The listing builds one solid part. Answer for the finished solid, in the listing's coordinates (mm). Give positions to 0.01 mm unless a question says otherwise; leave off trailing zeros. Write each loop counter-clockwise with the first axis right and the second up, starting at its lowest first coordinate (ties: lowest second). Pieces come first, ordered by that corner, then holes. Notation, with made-up numbers: (35.5, 12) - (65.5, 12) arc R22 ccw to (65.5, 39) - close; hole circle Ø3 at (51, 46). An arc over 180 degrees is marked (long way). Use a Markdown table: item, result. Add a question column.
from build123d import *

# Parameters (mm, degrees)
SKETCH1_W              = 220
SKETCH1_H              = 160
BOSS_EXTRUDE1_DEPTH    = 10
CHAMFER1_SIZE          = 10
M10X1_0_TAPPED_HOLE1_D = 9
M4X0_7_TAPPED_HOLE1_D  = 3.3


with BuildPart() as part:
    # Sketch1 → Boss-Extrude1 (new body)
    with BuildSketch(Plane(origin=(0, 0, 0), x_dir=(1, 0, 0), z_dir=(0, 1, 0))):
        Rectangle(SKETCH1_W, SKETCH1_H)
    extrude(amount=BOSS_EXTRUDE1_DEPTH)

    # Chamfer1
    chamfer1_edges = [part.edges().sort_by_distance(p)[0] for p in [
        (-110, 5, -80),
        (110, 5, -80),
        (110, 5, 80),
        (-110, 5, 80),
    ]]
    chamfer(chamfer1_edges, length=CHAMFER1_SIZE)

    # M10x1.0 Tapped Hole1 (through all)
    with Locations(Plane(origin=(0, 10, -55), x_dir=(0, 0, 1), z_dir=(0, 1, 0))):
        with Locations((0, 0), (110, -85), (110, 85)):
            Hole(M10X1_0_TAPPED_HOLE1_D / 2)

    # M4x0.7 Tapped Hole1 (through all)
    with Locations(Plane(origin=(30, 10, 0), x_dir=(0, 0, 1), z_dir=(0, 1, 0))):
        with Locations((0, 0)):
            m4x0_7_tapped_hole1 = Hole(M4X0_7_TAPPED_HOLE1_D / 2)

    # Mirror1: M4x0.7 Tapped Hole1 across plane
    add(m4x0_7_tapped_hole1.mirror(Plane(origin=(0, 0, 0), x_dir=(0, 0, 1), z_dir=(1, 0, 0))), mode=Mode.SUBTRACT)


solid = part.part
1. The part is cut by section B-B (x = -85). Give the vertices of the cut face in (y, z), and give its area (3 significant figures).
2. Consider L1, parallel to X at y = 4.25, z = 55; L2, parallel to X at y = 7.75, z = 0; L3, parallel to X at y = 2.75, z = -55. Determine where each line is inside the solid, lowest interval first. Write a range as [from, to].
3. For a pull along Z with two mould halves and no side action, classify faces 1 (the cylindrical face through (1.352, 4.93, -59.292)), 2 (the flat face through (-105, 5, 75)), 3 (the flat face through (105, 5, -75)) as released by +Z, released by -Z, zero draft, split by the parting line, or undercut.
4. The part is cut by section A-A (z = 55). Give the vertices of the cut face in (x, y).
Check values:
| question | item | result |
|---|---|---|
| 1 | outline | (0, -80) - (10, -80) - (10, 50.5) - (0, 50.5) - close; (0, 59.5) - (10, 59.5) - (10, 80) - (0, 80) - close |
| 1 | area | 1,510 mm2 |
| 2 | L1 | x = [-110, -89.5], [-80.5, 80.5], [89.5, 110] |
| 2 | L2 | x = [-110, -31.65], [-28.35, 28.35], [31.65, 110] |
| 2 | L3 | x = [-110, -4.5], [4.5, 110] |
| 3 | face 1 | undercut |
| 3 | face 2 | released by +Z |
| 3 | face 3 | released by -Z |
| 4 | outline | (-110, 0) - (-89.5, 0) - (-89.5, 10) - (-110, 10) - close; (-80.5, 0) - (80.5, 0) - (80.5, 10) - (-80.5, 10) - close; (89.5, 0) - (110, 0) - (110, 10) - (89.5, 10) - close |
